Autodesk Inventor part; units mm, degrees
ref_plane "YZ Plane" through (0, 0, 0) normal (1, 0, 0) x (0, 1, 0)
ref_plane "XZ Plane" through (0, 0, 0) normal (0, 1, 0) x (-1, 0, 0)
ref_plane "XY Plane" through (0, 0, 0) normal (0, 0, 1) x (1, 0, 0)
sketch "Sketch1" plane through (0, 0, 0) normal (0, 0, 1) x (1, 0, 0)
  line L0 (0, 31.5) -> (0, -31.5) construction
  line L1 (-31.5, 0) -> (31.5, 0) construction
  line L2 (-19.5, 19.5) -> (19.5, 19.5)
  line L3 (19.5, 19.5) -> (19.5, -19.5)
  line L4 (19.5, -19.5) -> (-19.5, -19.5)
  line L5 (-19.5, -19.5) -> (-19.5, 19.5)
  line L6 (-22.5, 22.5) -> (22.5, 22.5)
  line L7 (22.5, 22.5) -> (22.5, -22.5)
  line L8 (22.5, -22.5) -> (-22.5, -22.5)
  line L9 (-22.5, -22.5) -> (-22.5, 22.5)
  point P0 (0, 0)
  dimension "d0" = 39
  dimension "d1" = 39
  dimension "d2" = 3
  dimension "d3" = 3
  dimension "d4" = 3
  dimension "d5" = 3
extrude "Extrusion1" add sketch "Sketch1" along normal blind 40
sketch "Sketch2" plane through (0, 0, 0) normal (0, 0, -1) x (-1, 0, 0)
  line L0 (-22.5, -22.5) -> (22.5, -22.5)
  line L1 (22.5, -22.5) -> (22.5, 22.5)
  line L2 (22.5, 22.5) -> (-22.5, 22.5)
  line L3 (-22.5, 22.5) -> (-22.5, -22.5)
  point P0 (0, 0)
extrude "Extrusion2" add sketch "Sketch2" along normal blind 3
properties part number "Cuvette_45x45x40" material "Glass"
The model under review builds one solid part; all positions refer to its coordinate system, in mm. A direction names the side the tool comes from. Coordinates: 2 decimals unless noted, no trailing zeros. Order: outer loops, then holes, each group sorted by start corner. A loop starts at its lowest first (then second) coordinate and runs counter-clockwise, first axis right, second up. Notation, with made-up numbers: (28, -30) -> (43, -30) arc R35 cw to (43, 9) -> close; hole circle Ø6 at (-19, 70). An arc over 180 degrees is marked (long way). Answer in a Markdown table with one row per item. Add a question column.
Item 1: Machinability: for faces 1 (the flat face through (0, -22.5, 18)), 2 (the flat face through (19.5, 0, 20)), which of the approach directions +Z, -Z, +X, -X, +Y, -Y give a long, thin tool a straight path to every point of the face, cutting with its end or side? Answer none if there is none.
Item 2: To check wall thickness, follow probe 1 along Y at (x, z) = (-4, 15); probe 2 along Z at (x, y) = (-10, 5). State the ranges of each line that lie inside material, in increasing order.
Item 3: We need section A-A on z = 10.5. Write out the cut boundary in (x, y), plus the area to 3 significant figures.
Item 4: Mouldability with a two-part tool opening along X and no side actions: class faces 3 (the flat face through (0, 0, -3)), 4 (the flat face through (0, -19.5, 20)), 5 (the flat face through (22.5, 0, 18)) as +X half, -X half, draft (parallel to the pull), parting line (faces both ways), or undercut.
Item 5: Clearance check with a flat-ended pin moving along its axis: pin 1 (10 mm diameter, centred on x = 7, y = -1, fed in from +Z). State where the tip first meets the part, or that it passes through.
Item 6: We need section B-B on x = 11. Write out the cut boundary in (y, z), plus the area to 3 significant figures.
Final values:
| question | item | result |
|---|---|---|
| 1 | face 1 | +Z, -Z, +X, -X, -Y |
| 1 | face 2 | +Z |
| 2 | probe 1 | y = -22.5 to -19.5, 19.5 to 22.5 |
| 2 | probe 2 | z = -3 to 0 |
| 3 | outline | (-22.5, -22.5) -> (22.5, -22.5) -> (22.5, 22.5) -> (-22.5, 22.5) -> close; hole (-19.5, -19.5) -> (19.5, -19.5) -> (19.5, 19.5) -> (-19.5, 19.5) -> close |
| 3 | area | 504 mm2 |
| 4 | face 3 | draft |
| 4 | face 4 | undercut |
| 4 | face 5 | +X half |
| 5 | pin 1 | stops at z = 0 |
| 6 | outline | (-22.5, -3) -> (22.5, -3) -> (22.5, 40) -> (19.5, 40) -> (19.5, 0) -> (-19.5, 0) -> (-19.5, 40) -> (-22.5, 40) -> close |
| 6 | area | 375 mm2 |
